Job drawing, mm, ordinate dimensions from the low corner. One solid piece. Give positions to 0.01 mm unless a question says otherwise; leave off trailing zeros. Write each loop counter-clockwise with the first axis right and the second up, starting at its lowest first coordinate (ties: lowest second). Pieces come first, ordered by that corner, then holes. Notation, with made-up numbers: M 34.5,-39.75 L 82.5,-39.75 A14 cw 82.5,-24.75 Z; hole C -30.75,54.5 d8. An arc over 180 degrees is marked long. Use CSV: the item, a comma, the result in double quotes. Start each with the question number.
Item 1: Cut at B-B (x = 1.1). List the corners of the cut face in (y, z), then the cut area to 3 significant figures.
Item 2: Cut at A-A (z = 9). List the corners of the cut face in (x, y), then the cut area to 3 significant figures.
Item 3: Pin check, flat tips, straight feed: pin 1 (5 mm diameter, centred on y = 9, z = 32.5, fed in from -X); pin 2 (4 mm diameter, centred on y = 44, z = 32.5, fed in from -X); pin 3 (3.5 mm diameter, centred on y = 9, z = 9, fed in from -X). Stop position of each tip, or through.
Item 4: Cut at C-C (y = 44). List the corners of the cut face in (x, z).
Item 5: Drill centre lines: line 1 (Y direction, x = 4.4, z = 32.5); line 2 (Z direction, x = 3.75, y = 9); line 3 (Z direction, x = 3.9, y = 9). Where is each one in solid material? Low to high. Write a range as [from, to].
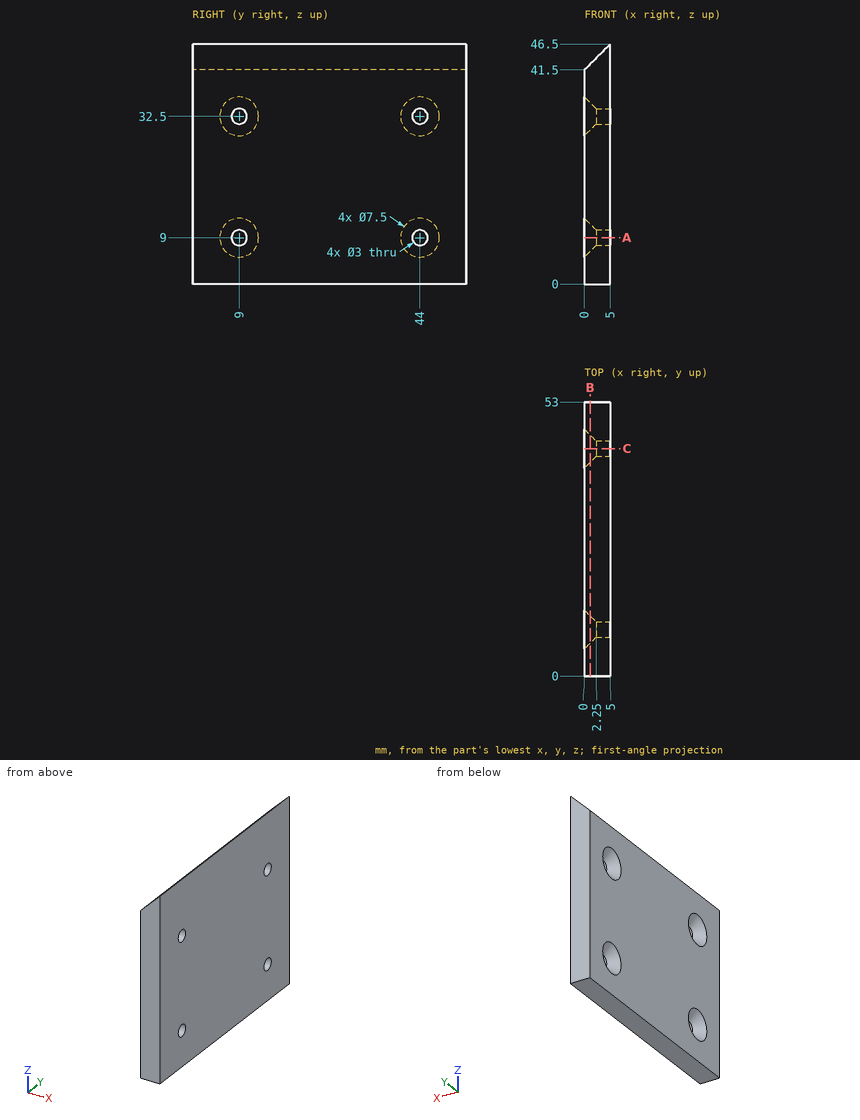
Worked answers:
1,outline,"M 0,0 L 53,0 L 53,42.6 L 0,42.6 Z; hole C 9,9 d5.3; hole C 9,32.5 d5.3; hole C 44,9 d5.3; hole C 44,32.5 d5.3"
1,area,"2,170 mm^2"
2,outline,"M 0,0 L 5,0 L 5,7.5 L 2.25,7.5 L 0,5.25 Z; M 0,12.75 L 2.25,10.5 L 5,10.5 L 5,42.5 L 2.25,42.5 L 0,40.25 Z; M 0,47.75 L 2.25,45.5 L 5,45.5 L 5,53 L 0,53 Z"
2,area,"225 mm^2"
3,pin 1,"stops at x = 1.25"
3,pin 2,"stops at x = 1.75"
3,pin 3,"stops at x = 2"
4,outline,"M 0,0 L 5,0 L 5,7.5 L 2.25,7.5 L 0,5.25 Z; M 0,12.75 L 2.25,10.5 L 5,10.5 L 5,31 L 2.25,31 L 0,28.75 Z; M 0,36.25 L 2.25,34 L 5,34 L 5,46.5 L 0,41.5 Z"
5,line 1,"y = [0, 7.5], [10.5, 42.5], [45.5, 53]"
5,line 2,"z = [0, 7.5], [10.5, 31], [34, 45.25]"
5,line 3,"z = [0, 7.5], [10.5, 31], [34, 45.4]"
